Build history of the part. All positions in model axes, mm. A direction names the side the tool comes from. Give positions to 0.01 mm unless a question says otherwise; leave off trailing zeros. Write each loop counter-clockwise with the first axis right and the second up, starting at its lowest first coordinate (ties: lowest second). Pieces come first, ordered by that corner, then holes. Notation, with made-up numbers: (-7.75, -40) -> (3.25, -40) arc R26 ccw to (3.25, -14) -> close; hole circle Ø3 at (65.25, -28). An arc over 180 degrees is marked (long way). Put each result on its own line as item: value.
Autodesk Inventor part; units mm, degrees
ref_plane "Work Plane1" through (32, 0, 0) normal (-1, 0, 0) x (0, 0, 1)
ref_plane "YZ Plane" through (0, 0, 0) normal (1, 0, 0) x (0, 1, 0)
ref_plane "XZ Plane" through (0, 0, 0) normal (0, 1, 0) x (-1, 0, 0)
sketch "Sketch1" plane through (0, 0, 0) normal (0, 0, 1) x (1, 0, 0)
  line L0 (0, 0) -> (23, 0)
  arc A0 (23, 0) -> (23, 18) centre (23, 9) ccw
  line L1 (23, 18) -> (0, 18)
  line L2 (0, 18) -> (0, 0)
  circle A1 centre (23, 9) radius 4.5
  dimension "d0" = 23
  dimension "d1" = 18
  dimension "d2" = 9
  dimension "d3" = 9
extrude "Extrusion1" add sketch "Sketch1" against normal blind 6
sketch "Sketch2" plane through (0, 18, 0) normal (0, 1, 0) x (1, 0, 0)
  circle A0 centre (18, 3) radius 1.5
  circle A1 centre (7, 3) radius 1.5
  point P0 (0, 0)
  dimension "d6" = 3
  dimension "d7" = 3
extrude "Extrusion2" cut sketch "Sketch2" against normal blind 5
sketch "Sketch3" plane through (0, 0, 0) normal (0, 0, 1) x (1, 0, 0)
  line L0 (20, 0) -> (26, 0)
  line L1 (26, 0) -> (26, 6)
  line L2 (26, 6) -> (20, 6)
  line L3 (20, 6) -> (20, 0)
  point P0 (0, 0)
  dimension "d10" = 6
  dimension "d11" = 6
extrude "Extrusion3" cut sketch "Sketch3" against normal through all
ref_plane "Work Plane1" through (32, 0, 0) normal (-1, 0, 0) x (0, 0, 1)
sketch "Sketch4" plane through (32, 0, 0) normal (-1, 0, 0) x (0, 0, 1)
  circle A0 centre (-3, 9) radius 1.5
  point P0 (0, 0)
  dimension "d15" = 3
extrude "Extrusion4" cut sketch "Sketch4" along normal blind 18
properties part number "Hand - Digit 2-3"
1) Slice it at C-C (z = -2). Write the cut outline in (x, y).
Filled sheet:
outline: (0, 0) -> (20, 0) -> (20, 5.65) arc R4.5 cw to (18.64, 7.88) -> (14, 7.88) -> (14, 10.12) -> (18.64, 10.12) arc R4.5 cw to (27.36, 10.12) -> (31.93, 10.12) arc R9 ccw to (23, 18) -> (19.12, 18) -> (19.12, 13) -> (16.88, 13) -> (16.88, 18) -> (8.12, 18) -> (8.12, 13) -> (5.88, 13) -> (5.88, 18) -> (0, 18) -> close; (26, 0.51) arc R9 ccw to (31.93, 7.88) -> (27.36, 7.88) arc R4.5 cw to (26, 5.65) -> close
2) Slice it at B-B (x = 18). Write the cut outline in (y, z).
Filled sheet:
outline: (0, -6) -> (18, -6) -> (18, -4.5) -> (13, -4.5) -> (13, -1.5) -> (18, -1.5) -> (18, 0) -> (0, 0) -> close; hole circle Ø3 at (9, -3)
3) Slice it at A-A (y = 9). Write the cut outline in (x, z).
Filled sheet:
outline: (0, -6) -> (18.5, -6) -> (18.5, -4.5) -> (14, -4.5) -> (14, -1.5) -> (18.5, -1.5) -> (18.5, 0) -> (0, 0) -> close; (27.5, -6) -> (32, -6) -> (32, -4.5) -> (27.5, -4.5) -> close; (27.5, -1.5) -> (32, -1.5) -> (32, 0) -> (27.5, 0) -> close
4) Wall check: L1, parallel to Z at x = 29.65, y = 9; L2, parallel to X at y = 16.25, z = -3.75; L3, parallel to X at y = 16.75, z = -2.75. Give the ranges that are in metal, low to high.
Filled sheet:
L1: -6 to -4.5, -1.5 to 0
L2: 0 to 5.7, 8.3 to 16.7, 19.3 to 28.33
L3: 0 to 5.52, 8.48 to 16.52, 19.48 to 27.58
5) Pull direction Z, two halves, no side cores. Call faces 5 (the flat face through (0, 9, -3)), 6 (the flat face through (12, 9, -6)), 7 (the cylindrical face through (29.65, 10.33, -2.31)): released by +Z, released by -Z, zero draft, split by the parting line, or undercut.
Filled sheet:
face 5: zero draft
face 6: released by -Z
face 7: undercut
6) Tool access for faces 1 (the flat face through (12, 9, 0)), 2 (the flat face through (14, 9, -3)), 3 (the flat face through (26, 3, -3)), 4 (the flat face through (18, 13, -3)): list every direction of +Z, -Z, +X, -X, +Y, -Y with a clear straight run to the whole face (end or side of a thin tool).
Filled sheet:
face 1: +Z, +X, -X, +Y, -Y
face 2: +X
face 3: +Z, -Z, -Y
face 4: +Y
7) Pin check, flat tips, straight feed: pin 1 (1.7 mm diameter, centred on y = 3.5, z = -4.5, fed in from +X); pin 2 (1.5 mm diameter, centred on x = 17.5, z = -3.5, fed in from +Y); pin 3 (2 mm diameter, centred on y = 13.5, z = -4.5, fed in from +X). Stop position of each tip, or through.
Filled sheet:
pin 1: x = 30.71
pin 2: y = 13
pin 3: x = 31.29
8) Slice it at D-D (y = 1.75). Write the cut outline in (x, z), plus the area to 3 significant figures.
Filled sheet:
outline: (0, -6) -> (20, -6) -> (20, 0) -> (0, 0) -> close; (26, -6) -> (28.33, -6) -> (28.33, 0) -> (26, 0) -> close
area: 134 mm2
